from build123d import *

# Parameters (mm, degrees)
SKETCH1_R               = 2.5
BOSS_EXTRUDE1_DEPTH     = 5
CUT_EXTRUDE1_REACH      = 41.937
CUT_EXTRUDE1_END_RADIUS = 2.5
SKETCH2_R               = 1.5
SKETCH3_R               = 2
CUT_EXTRUDE2_DEPTH      = 37.742346215


with BuildPart() as part:
    # Sketch1 → Boss-Extrude1 (new, symmetric)
    with BuildSketch(Plane.XY):
        with BuildLine():
            Line((0, 0), (29, 0))
            Line((29, 0), (29, 5))
            Line((29, 5), (20, 5))
            ThreePointArc((20, 5), (19.292893219, 5.292893219), (19, 6))
            Line((19, 6), (19, 27))
            Line((19, 27), (10, 27))
            Line((10, 27), (10, 6))
            ThreePointArc((10, 6), (9.707106781, 5.292893219), (9, 5))
            Line((9, 5), (0, 5))
            Line((0, 5), (0, 0))
        make_face()
        with Locations((14.5, 20)):
            Circle(SKETCH1_R, mode=Mode.SUBTRACT)
    extrude(amount=BOSS_EXTRUDE1_DEPTH, both=True)

    # Cut-Extrude1: up to this cylinder (the profile starts outside it)
    cut_extrude1_end = Plane(origin=(14.5, 20, 0), z_dir=(0, 0, -1)) * Cylinder(CUT_EXTRUDE1_END_RADIUS, 89.874, mode=Mode.PRIVATE)
    # Sketch2 → Cut-Extrude1 (cut, up to the surface)
    with BuildSketch(Plane(origin=(0, 27, 0), x_dir=(1, 0, 0), z_dir=(0, 1, 0)), mode=Mode.PRIVATE) as cut_extrude1_sk1:
        with Locations(Location((14.5, 0, 0), (0, 0, 270))):
            Circle(SKETCH2_R)
    cut_extrude1_tool1 = extrude(cut_extrude1_sk1.sketch, amount=-CUT_EXTRUDE1_REACH, mode=Mode.PRIVATE) - cut_extrude1_end
    add(cut_extrude1_tool1.solids().sort_by_distance((14.5, 27, 0))[0], mode=Mode.SUBTRACT)

    # Sketch3 → Cut-Extrude2 (cut, through all)
    with BuildSketch(Plane(origin=(0, 5, 0), x_dir=(1, 0, 0), z_dir=(0, 1, 0))):
        with Locations(Location((4.5, 0, 0), (0, 0, 180))):
            Circle(SKETCH3_R)
        with Locations(Location((24.5, 0, 0), (0, 0, 180))):
            Circle(SKETCH3_R)
    extrude(amount=-CUT_EXTRUDE2_DEPTH, mode=Mode.SUBTRACT)


solid = part.part
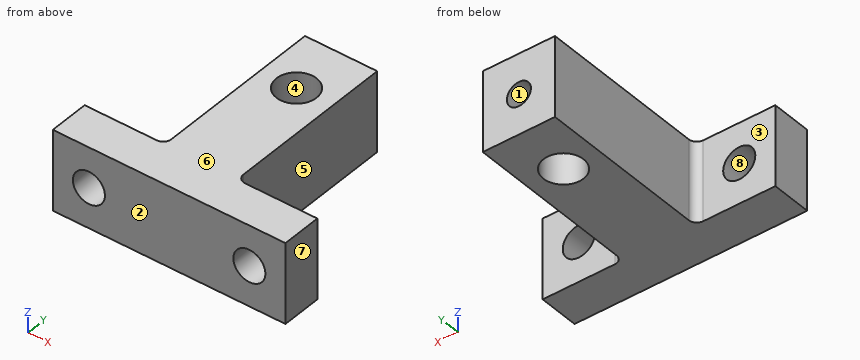
Verification items for the finished model (mm, model axes). Face numbers are marked on the shaded views. A direction names the side the tool comes from. Coordinates: 2 decimals unless noted, no trailing zeros. Write each loop counter-clockwise with the first axis right and the second up, starting at its lowest first coordinate (ties: lowest second). Pieces come first, ordered by that corner, then holes. Notation, with made-up numbers: (-28, 39.5) -> (-18, 39.5) arc R25 cw to (-18, 77.5) -> close; hole circle Ø5 at (37, 15). An arc over 180 degrees is marked (long way). One line per item, written item: value. Start each with the question number.
Q1. Cross-section at D-D on z = 0. Enter the section's corners in (x, y).
Q2. Cross-section at B-B on z = 3.25. Enter the section's corners in (x, y), and give its area (3 significant figures).
Q3. Mould release check, pull along Z, two halves, no side actions. Record for the marked faces 6, 7 and 8: pulls with the +Z half, pulls with the -Z half, needs draft (parallel to the pull), parting line crosses it, or undercut.
Q4. Cross-section at C-C on y = 2.5. Enter the section's corners in (x, z), and give its area (3 significant figures).
Q5. Access from +Z, -Z, +X, -X, +Y, -Y to the whole of each face (thin tool, end or side, straight path). Record for the marked faces 1, 2, 3, 4 and 5.
Q6. Thickness scan on L1, parallel to X at y = 24.15, z = 0; L2, parallel to Z at x = 4.5, y = 1.55; L3, parallel to X at y = 24.5, z = 2.25. Record the ranges inside material, lowest first. Write a range as from..to.
Q7. Cross-section at A-A on x = 14.5. Enter the section's corners in (y, z).
Q8. Go/stop test with flat-tipped pins: P1, Ø3, axis at y = 12.5, z = -1.5, coming from the -X side; P2, Ø5, axis at y = 13.5, z = 1.5, coming from the +X side; P3, Ø4.5, axis at x = 4, z = 0.5, coming from the +Y side. Record where each tip stops, or that it passes through.
Checked values:
1. outline: (0, 0) -> (2.5, 0) -> (2.5, 5) -> (0, 5) -> close; (6.5, 0) -> (22.5, 0) -> (22.5, 5) -> (20, 5) arc R1 cw to (19, 6) -> (19, 27) -> (16, 27) -> (16, 22) arc R2.5 cw (long way) to (13, 22) -> (13, 27) -> (10, 27) -> (10, 6) arc R1 cw to (9, 5) -> (6.5, 5) -> close; (26.5, 0) -> (29, 0) -> (29, 5) -> (26.5, 5) -> close
2. outline: (0, 0) -> (29, 0) -> (29, 5) -> (20, 5) arc R1 cw to (19, 6) -> (19, 27) -> (10, 27) -> (10, 6) arc R1 cw to (9, 5) -> (0, 5) -> close; hole circle Ø5 at (14.5, 20)
2. area: 324 mm²
3. face 6: pulls with the +Z half
3. face 7: needs draft
3. face 8: undercut
4. outline: (0, -5) -> (29, -5) -> (29, 5) -> (0, 5) -> close; hole circle Ø4 at (4.5, 0); hole circle Ø4 at (24.5, 0)
4. area: 265 mm²
5. face 1: +Y
5. face 2: +Z, -Z, +X, -X, -Y
5. face 3: +Z, -Z, -X, +Y
5. face 4: +Z, -Z
5. face 5: +Z, -Z, +X, +Y
6. L1: x = 10..13, 16..19
6. L2: z = -5..-2, 2..5
6. L3: x = 10..19
7. outline: (0, -5) -> (17.5, -5) -> (17.5, 5) -> (0, 5) -> close; (22.5, -5) -> (27, -5) -> (27, -1.5) -> (22.5, -1.5) -> close; (22.5, 1.5) -> (27, 1.5) -> (27, 5) -> (22.5, 5) -> close
8. P1: stops at x = 10
8. P2: stops at x = 19
8. P3: stops at y = 5
